```python
from build123d import *

# Parameters (mm, degrees)
SALIENTE_EXTRUIR1_DEPTH = 5
CROQUIS2_W              = 143
CROQUIS2_H              = 35
CORTAR_EXTRUIR1_DEPTH   = 5
REDONDEO1_R             = 10
CROQUIS3_W              = 5
CROQUIS3_H              = 8
SALIENTE_EXTRUIR2_DEPTH = 8
REDONDEO2_R             = 30
REDONDEO3_R             = 3
CROQUIS4_W              = 5.2
CROQUIS4_H              = 8.2
CORTAR_EXTRUIR2_DEPTH   = 192.034028382
REDONDEO4_R             = 3
REDONDEO5_R             = 10
REDONDEO6_R             = 1
CROQUIS5_R              = 1.5
CORTAR_EXTRUIR3_DEPTH   = 5
CROQUIS6_W              = 10.2
CROQUIS6_H              = 5.2
CORTAR_EXTRUIR4_DEPTH   = 5
CROQUIS7_W              = 132.4
CROQUIS7_H              = 10.8
CORTAR_EXTRUIR5_DEPTH   = 5
CROQUIS8_W              = 70
CROQUIS8_H              = 31
SALIENTE_EXTRUIR3_DEPTH = 5
CROQUIS9_W              = 8.2
CROQUIS9_H              = 5.2
CORTAR_EXTRUIR6_DEPTH   = 5
CROQUIS10_W             = 50
CROQUIS10_H             = 10.8
CORTAR_EXTRUIR7_DEPTH   = 5
REDONDEO9_R             = 3
REDONDEO10_R            = 6
REDONDEO11_R            = 5
REDONDEO12_R            = 5
CROQUIS12_W             = 22.569775484
CROQUIS12_H             = 11.5
CROQUIS12_W_2           = 25
CROQUIS12_H_2           = 3
SALIENTE_EXTRUIR4_DEPTH = 5
CORTAR_EXTRUIR8_DEPTH   = 5
REDONDEO8_R             = 3
REDONDEO13_R            = 1.2
REDONDEO14_R            = 15


with BuildPart() as part:
    # Croquis1 → Saliente-Extruir1 (new body)
    with BuildSketch(Plane.XY):
        Polygon((0, 0), (0, 70), (125, 70), (150, 87), (160, 87), (170, 70), (170, 0), align=None)
    extrude(amount=SALIENTE_EXTRUIR1_DEPTH)

    # Croquis2 → Cortar-Extruir1 (cut)
    with BuildSketch(Plane.XY.offset(5)):
        with Locations((83.5, 17.5)):
            Rectangle(CROQUIS2_W, CROQUIS2_H)
    extrude(amount=-CORTAR_EXTRUIR1_DEPTH, mode=Mode.SUBTRACT)

    # Redondeo1
    redondeo1_edges = [part.edges().sort_by_distance(p)[0] for p in [
        (12, 35, 2.5),
        (155, 35, 2.5),
    ]]
    fillet(redondeo1_edges, radius=REDONDEO1_R)

    # Croquis3 → Saliente-Extruir2 (add)
    with BuildSketch(Plane.ZY):
        with Locations((2.5, 15)):
            Rectangle(CROQUIS3_W, CROQUIS3_H)
        with Locations((2.5, 55)):
            Rectangle(CROQUIS3_W, CROQUIS3_H)
    extrude(amount=SALIENTE_EXTRUIR2_DEPTH)

    # Redondeo2
    redondeo2_edges = [part.edges().sort_by_distance(p)[0] for p in [
        (125, 70, 2.5),
        (170, 70, 2.5),
    ]]
    fillet(redondeo2_edges, radius=REDONDEO2_R)

    # Redondeo3
    redondeo3_edges = [part.edges().sort_by_distance(p)[0] for p in [
        (170, 0, 2.5),
        (12, 0, 2.5),
        (155, 0, 2.5),
    ]]
    fillet(redondeo3_edges, radius=REDONDEO3_R)

    # Croquis4 → Cortar-Extruir2 (cut, through all)
    with BuildSketch(Plane.XY.offset(5)):
        with Locations((155, 78)):
            Rectangle(CROQUIS4_W, CROQUIS4_H)
        with Locations((155, 54)):
            Rectangle(CROQUIS4_W, CROQUIS4_H)
    extrude(amount=-CORTAR_EXTRUIR2_DEPTH, mode=Mode.SUBTRACT)

    # Redondeo4
    redondeo4_edges = [part.edges().sort_by_distance(p)[0] for p in [
        (160, 87, 2.5),
    ]]
    fillet(redondeo4_edges, radius=REDONDEO4_R)

    # Redondeo5
    redondeo5_edges = [part.edges().sort_by_distance(p)[0] for p in [
        (150, 87, 2.5),
    ]]
    fillet(redondeo5_edges, radius=REDONDEO5_R)

    # Redondeo6
    redondeo6_edges = [part.edges().sort_by_distance(p)[0] for p in [
        (-8, 19, 2.5),
        (-8, 11, 2.5),
        (-8, 59, 2.5),
        (-8, 51, 2.5),
    ]]
    fillet(redondeo6_edges, radius=REDONDEO6_R)

    # Croquis5 → Cortar-Extruir3 (cut)
    with BuildSketch(Plane.XY.offset(5)):
        with Locations((-4, 55)):
            Circle(CROQUIS5_R)
        with Locations((-4, 15)):
            Circle(CROQUIS5_R)
    extrude(amount=-CORTAR_EXTRUIR3_DEPTH, mode=Mode.SUBTRACT)

    # Croquis6 → Cortar-Extruir4 (cut)
    with BuildSketch(Plane.XY.offset(5)):
        with Locations((80, 42.6)):
            Rectangle(CROQUIS6_W, CROQUIS6_H)
        with Locations((30, 42.6)):
            Rectangle(CROQUIS6_W, CROQUIS6_H)
        with Locations((130, 42.6)):
            Rectangle(CROQUIS6_W, CROQUIS6_H)
    extrude(amount=-CORTAR_EXTRUIR4_DEPTH, mode=Mode.SUBTRACT)

    # Croquis7 → Cortar-Extruir5 (cut)
    with BuildSketch(Plane.XY.offset(5)):
        with Locations((76.2, 57.6)):
            Rectangle(CROQUIS7_W, CROQUIS7_H)
    extrude(amount=-CORTAR_EXTRUIR5_DEPTH, mode=Mode.SUBTRACT)

    # Croquis8 → Saliente-Extruir3 (add)
    with BuildSketch(Plane.XY.offset(5)):
        with Locations((55, 85.5)):
            Rectangle(CROQUIS8_W, CROQUIS8_H)
    extrude(amount=-SALIENTE_EXTRUIR3_DEPTH)

    # Croquis9 → Cortar-Extruir6 (cut)
    with BuildSketch(Plane.XY.offset(5)):
        with Locations((35, 93.4)):
            Rectangle(CROQUIS9_W, CROQUIS9_H)
        with Locations((75, 93.4)):
            Rectangle(CROQUIS9_W, CROQUIS9_H)
    extrude(amount=-CORTAR_EXTRUIR6_DEPTH, mode=Mode.SUBTRACT)

    # Croquis10 → Cortar-Extruir7 (cut)
    with BuildSketch(Plane.XY.offset(5)):
        with Locations((55, 77.4)):
            Rectangle(CROQUIS10_W, CROQUIS10_H)
    extrude(amount=-CORTAR_EXTRUIR7_DEPTH, mode=Mode.SUBTRACT)

    # Redondeo9
    redondeo9_edges = [part.edges().sort_by_distance(p)[0] for p in [
        (30, 72, 2.5),
        (30, 82.8, 2.5),
        (80, 82.8, 2.5),
        (80, 72, 2.5),
    ]]
    fillet(redondeo9_edges, radius=REDONDEO9_R)

    # Redondeo10
    redondeo10_edges = [part.edges().sort_by_distance(p)[0] for p in [
        (20, 70, 2.5),
        (90, 70, 2.5),
    ]]
    fillet(redondeo10_edges, radius=REDONDEO10_R)

    # Redondeo11
    redondeo11_edges = [part.edges().sort_by_distance(p)[0] for p in [
        (20, 101, 2.5),
        (90, 101, 2.5),
    ]]
    fillet(redondeo11_edges, radius=REDONDEO11_R)

    # Redondeo12
    redondeo12_edges = [part.edges().sort_by_distance(p)[0] for p in [
        (0, 70, 2.5),
    ]]
    fillet(redondeo12_edges, radius=REDONDEO12_R)

    # Croquis12 → Saliente-Extruir4 (add)
    with BuildSketch(Plane.XY.offset(5)):
        with Locations((120.284887742, 68.75)):
            Rectangle(CROQUIS12_W, CROQUIS12_H)
        with Locations((121.5, 53.7)):
            Rectangle(CROQUIS12_W_2, CROQUIS12_H_2)
    extrude(amount=-SALIENTE_EXTRUIR4_DEPTH)

    # Croquis11 → Cortar-Extruir8 (cut)
    with BuildSketch(Plane.XY.offset(5)):
        with BuildLine():
            Line((129, 48.45), (114, 48.45))
            ThreePointArc((114, 48.45), (112.25, 50.2), (114, 51.95))
            Line((114, 51.95), (129, 51.95))
            ThreePointArc((129, 51.95), (130.75, 50.2), (129, 48.45))
        make_face()
        with BuildLine():
            Line((129, 67.45), (114, 67.45))
            ThreePointArc((114, 67.45), (112.25, 69.2), (114, 70.95))
            Line((114, 70.95), (129, 70.95))
            ThreePointArc((129, 70.95), (130.75, 69.2), (129, 67.45))
        make_face()
    extrude(amount=-CORTAR_EXTRUIR8_DEPTH, mode=Mode.SUBTRACT)

    # Redondeo8
    redondeo8_edges = [part.edges().sort_by_distance(p)[0] for p in [
        (10, 52.2, 2.5),
        (10, 63, 2.5),
        (142.4, 63, 2.5),
        (142.4, 52.2, 2.5),
    ]]
    fillet(redondeo8_edges, radius=REDONDEO8_R)

    # Redondeo13
    redondeo13_edges = [part.edges().sort_by_distance(p)[0] for p in [
        (109, 70, 2.5),
        (109, 74.5, 2.5),
        (134, 55.2, 2.5),
        (134, 52.2, 2.5),
        (109, 52.2, 2.5),
        (109, 55.2, 2.5),
    ]]
    fillet(redondeo13_edges, radius=REDONDEO13_R)

    # Redondeo14
    redondeo14_edges = [part.edges().sort_by_distance(p)[0] for p in [
        (131.569775484, 74.5, 2.5),
    ]]
    fillet(redondeo14_edges, radius=REDONDEO14_R)


solid = part.part
```
Could you check a few things on this model? Use its own coordinates, in mm. A direction names the side the tool comes from. Give positions to 0.01 mm unless a question says otherwise; leave off trailing zeros. Loops run counter-clockwise (first coordinate to the right, second up) from the corner with the lowest first, then second, coordinate; pieces in that order, holes last. Notation, with made-up numbers: (16, 36) - (47, 36) arc R13 ccw to (47, 52) - close; hole circle Ø11 at (49, 72.25). An arc over 180 degrees is marked (long way). Answer in a Markdown table with one row per item. Add a question column.
Q1. If we section it at A-A (y = 21): List the corners of the cut face in (x, z) for me, plus the area to 3 significant figures.
Q2. Which directions (+Z, -Z, +X, -X, +Y, -Y) give clear straight access to the entire face, cutting with the end or side of a thin tool? Please do faces 5 (the face through (30, 77, 3)), 6 (the face through (0, 5, 2)), 7 (the face through (0, 62, 2)).
Q3. Please list where these lines run through material, in increasing order: L1, parallel to Y at x = -4, z = 2.15; L2, parallel to Y at x = 59.5, z = 3; L3, parallel to X at y = 58, z = 3.55. Write a range as from..to.
Q4. For pin 1 (2.5 mm diameter, centred on y = 72, z = 3, fed in from -X); pin 2 (2.5 mm diameter, centred on x = 103, z = 2.5, fed in from +Y); pin 3 (1.5 mm diameter, centred on y = 84.5, z = 2.5, fed in from -X), each with a flat end and sliding along its axis, tell me the tip position at first contact or that it passes through.
Q5. If we section it at C-C (z = 3.35): State how many separate pieces and enclosed holes the cut face has, plus the area to 3 significant figures.
Q6. If we section it at B-B (x = 64.5): List the corners of the cut face in (y, z) for me.
Q7. We'd pull the mould along Y, two halves only. Please class faces 1 (the face through (90, 86, 3)), 2 (the face through (150.18, 86.57, 2.54)), 3 (the face through (157.6, 78, 3)), 4 (the face through (121, 70.95, 3)): +Y half, -Y half, draft (parallel to the pull), parting line (faces both ways), or undercut.
The answers:
| question | item | result |
|---|---|---|
| 1 | outline | (0, 0) - (12, 0) - (12, 5) - (0, 5) - close; (155, 0) - (170, 0) - (170, 5) - (155, 5) - close |
| 1 | area | 135 mm^2 |
| 2 | face 5 | +Z, -Z |
| 2 | face 6 | +Z, -Z, -X, -Y |
| 2 | face 7 | +Z, -Z, -X, +Y |
| 3 | L1 | y = 11..13.5, 16.5..19, 51..53.5, 56.5..59 |
| 3 | L2 | y = 35..52.2, 63..72, 82.8..101 |
| 3 | L3 | x = -8..10, 142.4..152.4, 157.6..170 |
| 4 | pin 1 | stops at x = 16.9 |
| 4 | pin 2 | stops at y = 70 |
| 4 | pin 3 | stops at x = 20 |
| 5 | separate pieces | 1 |
| 5 | enclosed holes | 13 |
| 5 | area | 7,430 mm^2 |
| 6 | outline | (35, 0) - (52.2, 0) - (52.2, 5) - (35, 5) - close; (63, 0) - (72, 0) - (72, 5) - (63, 5) - close; (82.8, 0) - (101, 0) - (101, 5) - (82.8, 5) - close |
| 7 | face 1 | draft |
| 7 | face 2 | +Y half |
| 7 | face 3 | undercut |
| 7 | face 4 | undercut |
